Read the model definition and answer for the solid it produces. Units are mm, in the model's axes. A direction names the side the tool comes from. Coordinates: 2 decimals unless noted, no trailing zeros. Order: outer loops, then holes, each group sorted by start corner. A loop starts at its lowest first (then second) coordinate and runs counter-clockwise, first axis right, second up. Notation, with made-up numbers: M 82,24.5 L 94,24.5 A20 cw 94,48.5 Z; hole C 6,42.25 d1. An arc over 180 degrees is marked long. Use a Markdown table: item, result. Add a question column.
1) Find the intervals of material crossed by probe 1 along X at (y, z) = (0.25, 3) (3 decimals); probe 2 along Z at (x, y) = (0.5, 0.5); probe 3 along Y at (x, z) = (-2, -2.5), in increasing order. Write a range as [from, to].
2) The mould has two halves that part along X. Classify faces 1 (the face through (2.525, 2, 0)), 2 (the face through (0, 2, -47.5)), 3 (the face through (2.4, -3, 0)): released by +X, released by -X, zero draft, split by the parting line, or undercut.
3) Find section D-D on z = 26. Write down the section's boundary in (x, y) (3 decimals), plus the area to 4 significant figures.
4) Find section C-C on x = -0.75. Write down the section's boundary in (y, z), plus the area to 3 significant figures.
5) Find section A-A on z = 6. Write down the section's boundary in (x, y) (3 decimals).
6) For faces 4 (the face through (0, -2, -25)), 5 (the face through (-2.4, -3, 0)), 6 (the face through (0, 1, -25)), determine the directions among +Z, -Z, +X, -X, +Y, -Y from which every point of the face is accessible in a straight line to the end or side of a thin tool.
7) Each of these flat-tipped pins is pushed along its axis until it touches: pin 1 Ø2.5 at (x, z) = (-0.5, -6) entering from +Y; pin 2 Ø1 at (x, z) = (2, -24) entering from -Y; pin 3 Ø1.5 at (y, z) = (-4.5, 9.5) entering from +X; pin 4 Ø6 at (y, z) = (-1.5, 12.5) entering from +X. Where does it stop, or does it pass through?
8) Find section B-B on y = 4. Write down the section's boundary in (x, z) (3 decimals).
from build123d import *

# Parameters (mm, degrees)
SKETCH1_W           = 8
SKETCH1_H           = 95
SKETCH1_W_2         = 5.05
SKETCH1_H_2         = 50
BOSS_EXTRUDE1_DEPTH = 5
SKETCH1_2_W         = 8
SKETCH1_2_H         = 95
SKETCH1_2_W_2       = 5.05
SKETCH1_2_H_2       = 50
BOSS_EXTRUDE2_DEPTH = 1
SKETCH2_W           = 4.8
SKETCH2_H           = 50
BOSS_EXTRUDE3_DEPTH = 5
CHAMFER2_SIZE       = 2


with BuildPart() as part:
    # Sketch1 → Boss-Extrude1 (new body)
    with BuildSketch(Plane(origin=(0, 0, 0), x_dir=(1, 0, 0), z_dir=(0, 1, 0))):
        Rectangle(SKETCH1_W, SKETCH1_H)
        Rectangle(SKETCH1_W_2, SKETCH1_H_2, mode=Mode.SUBTRACT)
    extrude(amount=BOSS_EXTRUDE1_DEPTH)

    # Sketch1_2 → Boss-Extrude2 (add)
    with BuildSketch(Plane(origin=(0, 0, 0), x_dir=(1, 0, 0), z_dir=(0, 1, 0))):
        Rectangle(SKETCH1_2_W, SKETCH1_2_H)
        Rectangle(SKETCH1_2_W_2, SKETCH1_2_H_2, mode=Mode.SUBTRACT)
        Rectangle(SKETCH1_2_W_2, SKETCH1_2_H_2)
    extrude(amount=-BOSS_EXTRUDE2_DEPTH)

    # Sketch2 → Boss-Extrude3 (add)
    with BuildSketch(Plane.XZ.offset(1)):
        Rectangle(SKETCH2_W, SKETCH2_H)
    extrude(amount=BOSS_EXTRUDE3_DEPTH)

    # Chamfer2
    chamfer2_edges = [part.edges().sort_by_distance(p)[0] for p in [
        (0, 5, -25),
        (0, 5, 25),
        (0, -6, -25),
        (0, -6, 25),
    ]]
    chamfer(chamfer2_edges, length=CHAMFER2_SIZE)


solid = part.part
Check result:
| question | item | result |
|---|---|---|
| 1 | probe 1 | x = [-4, -2.525], [2.525, 4] |
| 1 | probe 2 | z = [-47.5, -25], [25, 47.5] |
| 1 | probe 3 | y = [-6, 0] |
| 2 | face 1 | undercut |
| 2 | face 2 | zero draft |
| 2 | face 3 | released by +X |
| 3 | outline | M -4,-1 L 4,-1 L 4,5 L 2.525,5 L 2.525,4 L -2.525,4 L -2.525,5 L -4,5 Z |
| 3 | area | 42.95 mm2 |
| 4 | outline | M -6,-23 L -4,-25 L -1,-25 L -1,-47.5 L 5,-47.5 L 5,-27 L 3,-25 L 0,-25 L 0,25 L 3,25 L 5,27 L 5,47.5 L -1,47.5 L -1,25 L -4,25 L -6,23 Z |
| 4 | area | 562 mm2 |
| 5 | outline | M -4,-1 L -2.4,-1 L -2.4,-6 L 2.4,-6 L 2.4,-1 L 4,-1 L 4,5 L 2.525,5 L 2.525,0 L -2.525,0 L -2.525,5 L -4,5 Z |
| 6 | face 4 | -Z, +X, -X, -Y |
| 6 | face 5 | +Z, -Z, -X, -Y |
| 6 | face 6 | +Y |
| 7 | pin 1 | stops at y = 0 |
| 7 | pin 2 | stops at y = -5.5 |
| 7 | pin 3 | stops at x = 2.4 |
| 7 | pin 4 | stops at x = 4 |
| 8 | outline | M -4,-47.5 L 4,-47.5 L 4,47.5 L -4,47.5 Z; hole M -2.525,-26 L 2.525,-26 L 2.525,26 L -2.525,26 Z |
